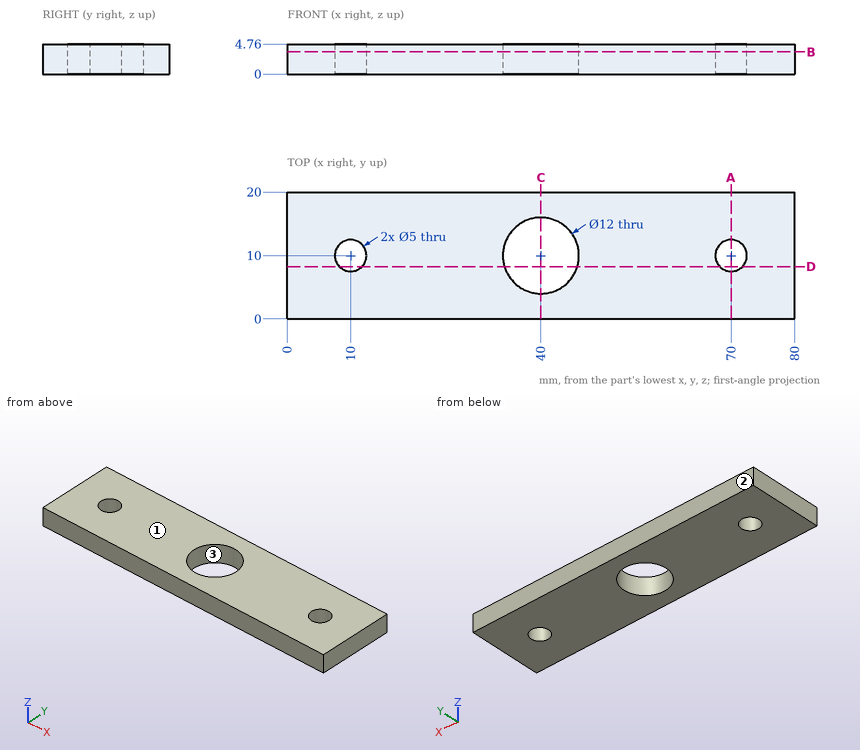
Check sheet for the drawn part. Datum: minimum x, y, z corner. Units: mm. Give positions to 0.01 mm unless a question says otherwise; leave off trailing zeros. Write each loop counter-clockwise with the first axis right and the second up, starting at its lowest first coordinate (ties: lowest second). Pieces come first, ordered by that corner, then holes. Notation, with made-up numbers: (-27, 78) - (31, 78) arc R29 cw to (31, 102) - close; hole circle Ø2 at (-27, 70.5). An arc over 180 degrees is marked (long way). Put each result on its own line as item: value.
1. Draft check along Y on the marked faces 1, 2 and 3. Enter one of: +Y half, -Y half, draft (parallel to the pull), parting line (faces both ways), or undercut.
Ans:
face 1: draft
face 2: +Y half
face 3: undercut
2. Thickness scan on line 1 (X direction, y = 10, z = 2.1); line 2 (Y direction, x = 10, z = 1.45); line 3 (Y direction, x = 11, z = 1). Record the ranges inside material, lowest first.
Ans:
line 1: x = 0 to 7.5, 12.5 to 34, 46 to 67.5, 72.5 to 80
line 2: y = 0 to 7.5, 12.5 to 20
line 3: y = 0 to 7.71, 12.29 to 20
3. Sectioned sample at C-C, the plane x = 40. Enter the section's corners in (y, z), plus the area to 3 significant figures.
Ans:
outline: (0, 0) - (4, 0) - (4, 4.76) - (0, 4.76) - close; (16, 0) - (20, 0) - (20, 4.76) - (16, 4.76) - close
area: 38.1 mm²
4. Sectioned sample at B-B, the plane z = 3.5. Enter the section's corners in (x, y), plus the area to 3 significant figures.
Ans:
outline: (0, 0) - (80, 0) - (80, 20) - (0, 20) - close; hole circle Ø5 at (10, 10); hole circle Ø12 at (40, 10); hole circle Ø5 at (70, 10)
area: 1,450 mm²
5. Sectioned sample at A-A, the plane x = 70. Enter the section's corners in (y, z), plus the area to 3 significant figures.
Ans:
outline: (0, 0) - (7.5, 0) - (7.5, 4.76) - (0, 4.76) - close; (12.5, 0) - (20, 0) - (20, 4.76) - (12.5, 4.76) - close
area: 71.4 mm²
6. Sectioned sample at D-D, the plane y = 8.25. Enter the section's corners in (x, z).
Ans:
outline: (0, 0) - (8.21, 0) - (8.21, 4.76) - (0, 4.76) - close; (11.79, 0) - (34.26, 0) - (34.26, 4.76) - (11.79, 4.76) - close; (45.74, 0) - (68.21, 0) - (68.21, 4.76) - (45.74, 4.76) - close; (71.79, 0) - (80, 0) - (80, 4.76) - (71.79, 4.76) - close
